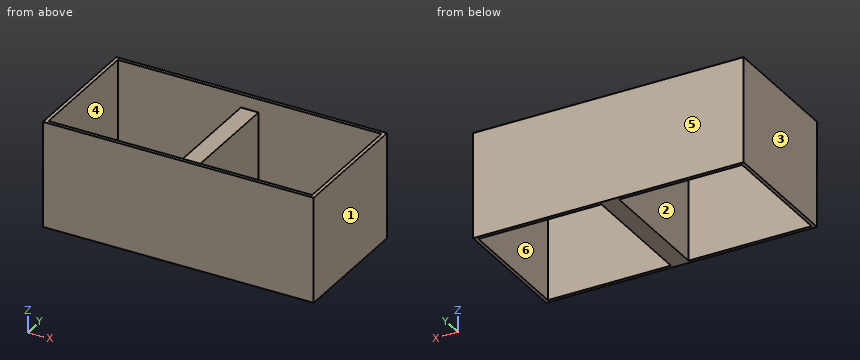
```python
from build123d import *

# Parameters (mm, degrees)
F1_W     = 782
F1_H     = 375.6
F2_DEPTH = 304.8
F0_W     = 762
F0_H     = 355.6
F3_DEPTH = 304.801
F4_W     = 50.8
F4_H     = 355.6
F5_DEPTH = 266.7


with BuildPart() as f2:
    # F1 (on Top) → F2 (new body)
    with BuildSketch(Plane.XY):
        with Locations((381, 177.8)):
            Rectangle(F1_W, F1_H)
    extrude(amount=F2_DEPTH)

    # F0 (on Top) → F3 (cut, through all)
    with BuildSketch(Plane.XY):
        with Locations((381, 177.8)):
            Rectangle(F0_W, F0_H)
    extrude(amount=F3_DEPTH, mode=Mode.SUBTRACT)

    # F4 (on face) → F5 (join)
    with BuildSketch(Plane(origin=(0, 0, 0), x_dir=(1, 0, 0), z_dir=(0, 0, -1))):
        with Locations((381, -177.8)):
            Rectangle(F4_W, F4_H)
    extrude(amount=-F5_DEPTH)


solid = f2.part
```
The listing builds one solid part. Answer for the finished solid, in the listing's coordinates (mm). Face numbers are marked on the shaded views. A direction names the side the tool comes from. Coordinates: 2 decimals unless noted, no trailing zeros. Write each loop counter-clockwise with the first axis right and the second up, starting at its lowest first coordinate (ties: lowest second). Pieces come first, ordered by that corner, then holes. Notation, with made-up numbers: (83.5, -28) - (91.5, -28) arc R37 ccw to (91.5, 11) - close; hole circle Ø4 at (-9.75, 4). An arc over 180 degrees is marked (long way). Return JSON: item names as keys, results as strings. Group by question number.
1. A cutting plane is placed at C-C, the plane z = 121.5. Determine the outline of the cut face in (x, y), plus the area to 3 significant figures.
2. Determine the mould class of the marked faces 3, 4, 5 and 6 for opening direction X: released by +X, released by -X, zero draft, split by the parting line, or undercut.
3. Straight lines are drawn through the part: L1, parallel to X at y = 54, z = 226; L2, parallel to Y at x = 543, z = 98.5; L3, parallel to Z at x = 372.5, y = 169. For each, find the intervals that lie inside material, in ascending order.
4. A cutting plane is placed at A-A, the plane x = 649. Determine the outline of the cut face in (y, z).
5. Which of the six approach directions +Z, -Z, +X, -X, +Y, -Y give full straight-line access (tool end or side, diameter ignored) to the marked faces 1 and 2?
6. A cutting plane is placed at B-B, the plane y = 324. Determine the outline of the cut face in (x, z), plus the area to 3 significant figures.
Ans:
{
 "1": {"outline": "(-10, -10) - (772, -10) - (772, 365.6) - (-10, 365.6) - close; hole (0, 0) - (355.6, 0) - (355.6, 355.6) - (0, 355.6) - close; hole (406.4, 0) - (762, 0) - (762, 355.6) - (406.4, 355.6) - close", "area": "40,800 mm²"},
 "2": {"face 3": "released by -X", "face 4": "undercut", "face 5": "zero draft", "face 6": "undercut"},
 "3": {"L1": "-10 to 0, 355.6 to 406.4, 762 to 772", "L2": "-10 to 0, 355.6 to 365.6", "L3": "0 to 266.7"},
 "4": {"outline": "(-10, 0) - (0, 0) - (0, 304.8) - (-10, 304.8) - close; (355.6, 0) - (365.6, 0) - (365.6, 304.8) - (355.6, 304.8) - close"},
 "5": {"face 1": "+Z, -Z, +X, +Y, -Y", "face 2": "+Z, -Z"},
 "6": {"outline": "(-10, 0) - (0, 0) - (0, 304.8) - (-10, 304.8) - close; (355.6, 0) - (406.4, 0) - (406.4, 266.7) - (355.6, 266.7) - close; (762, 0) - (772, 0) - (772, 304.8) - (762, 304.8) - close", "area": "19,600 mm²"}
}
